```python
from build123d import *

# Parameters (mm, degrees)
F2_R     = 5
F3_R     = 25
F4_DEPTH = 10


with BuildPart() as f1:
    # F0 (on Front) → F1 (revolve)
    with BuildSketch(Plane.XZ):
        Polygon((-60.746692, 14), (-60.746692, 0), (-45, 0), (-45, -32), (-21.65, -32), (-21.65, 27), (-45, 27), (-45, 14), align=None)
    revolve(axis=Axis((0, 0, 28.312229), (0, 0, 1)))

    # F2
    f2_edges = [f1.edges().sort_by_distance(p)[0] for p in [
        (45, 0, 27),
    ]]
    fillet(f2_edges, radius=F2_R)

    # F3 (on face) → F4 (cut)
    with BuildSketch(Plane(origin=(0, 0, -32), x_dir=(1, 0, 0), z_dir=(0, 0, -1))):
        Circle(F3_R)
    extrude(amount=-F4_DEPTH, mode=Mode.SUBTRACT)


solid = f1.part
```
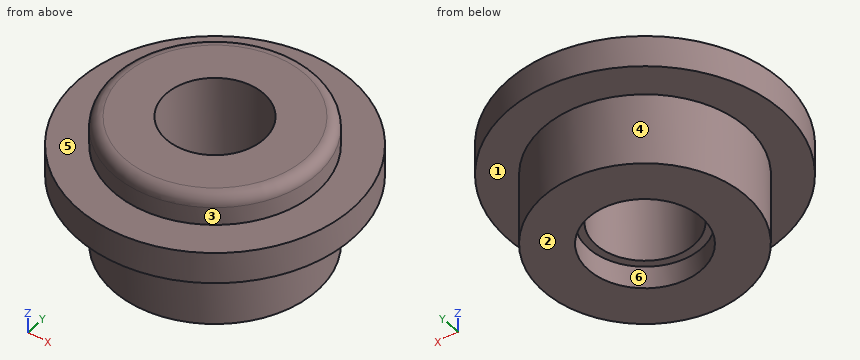
Can you work these out from the model? Positions are in its coordinate system, mm. Face numbers are marked on the shaded views. A direction names the side the tool comes from. Give positions to 0.01 mm unless a question says otherwise; leave off trailing zeros. Write each loop counter-clockwise with the first axis right and the second up, starting at its lowest first coordinate (ties: lowest second). Pieces come first, ordered by that corner, then holes. Notation, with made-up numbers: (32, -13.5) -> (54, -13.5) arc R16 cw to (54, 13.5) -> close; hole circle Ø10 at (-10.75, -36). An arc over 180 degrees is marked (long way). One line per item, written item: value.
Q1. Imagine slicing it at A-A on x = 0. Please give me the cut outline in (y, z).
Results found:
outline: (-60.75, 0) -> (-45, 0) -> (-45, -32) -> (-25, -32) -> (-25, -22) -> (-21.65, -22) -> (-21.65, 27) -> (-40, 27) arc R5 ccw to (-45, 22) -> (-45, 14) -> (-60.75, 14) -> close; (21.65, -22) -> (25, -22) -> (25, -32) -> (45, -32) -> (45, 0) -> (60.75, 0) -> (60.75, 14) -> (45, 14) -> (45, 22) arc R5 ccw to (40, 27) -> (21.65, 27) -> close
Q2. For P1, Ø3, axis at x = 36, y = 38, coming from the -Z side; P2, Ø5, axis at x = 10, z = -25.5, coming from the +Y side; P3, Ø4, axis at x = -23.5, z = -3, coming from the -Y side, each with a flat end and sliding along its axis, tell me the tip position at first contact or that it passes through.
Results found:
P1: stops at z = 0
P2: stops at y = 44.37
P3: stops at y = -39.53
Q3. We'd pull the mould along X, two halves only. Please class the marked faces 4, 5 and 6: +X half, -X half, draft (parallel to the pull), parting line (faces both ways), or undercut.
Results found:
face 4: parting line
face 5: draft
face 6: undercut
Q4. Imagine slicing it at D-D on z = -27. Please give me the cut outline in (x, y).
Results found:
outline: circle Ø90 at (0, 0); hole circle Ø50 at (0, 0)
Q5. Please list where these lines run through material, in increasing order: line 1 (X direction, y = 0, z = -24); line 2 (X direction, y = 0, z = 17). Write a range as [from, to].
Results found:
line 1: x = [-45, -25], [25, 45]
line 2: x = [-45, -21.65], [21.65, 45]
Q6. Which directions (+Z, -Z, +X, -X, +Y, -Y) give clear straight access to the entire face, cutting with the end or side of a thin tool? Please do the marked faces 1, 2 and 3.
Results found:
face 1: -Z
face 2: -Z, +X, -X, +Y, -Y
face 3: +Z
Q7. Imagine slicing it at C-C on z = -9. Please give me the cut outline in (x, y), and give its area (3 significant figures).
Results found:
outline: circle Ø90 at (0, 0); hole circle Ø43.3 at (0, 0)
area: 4,890 mm^2
